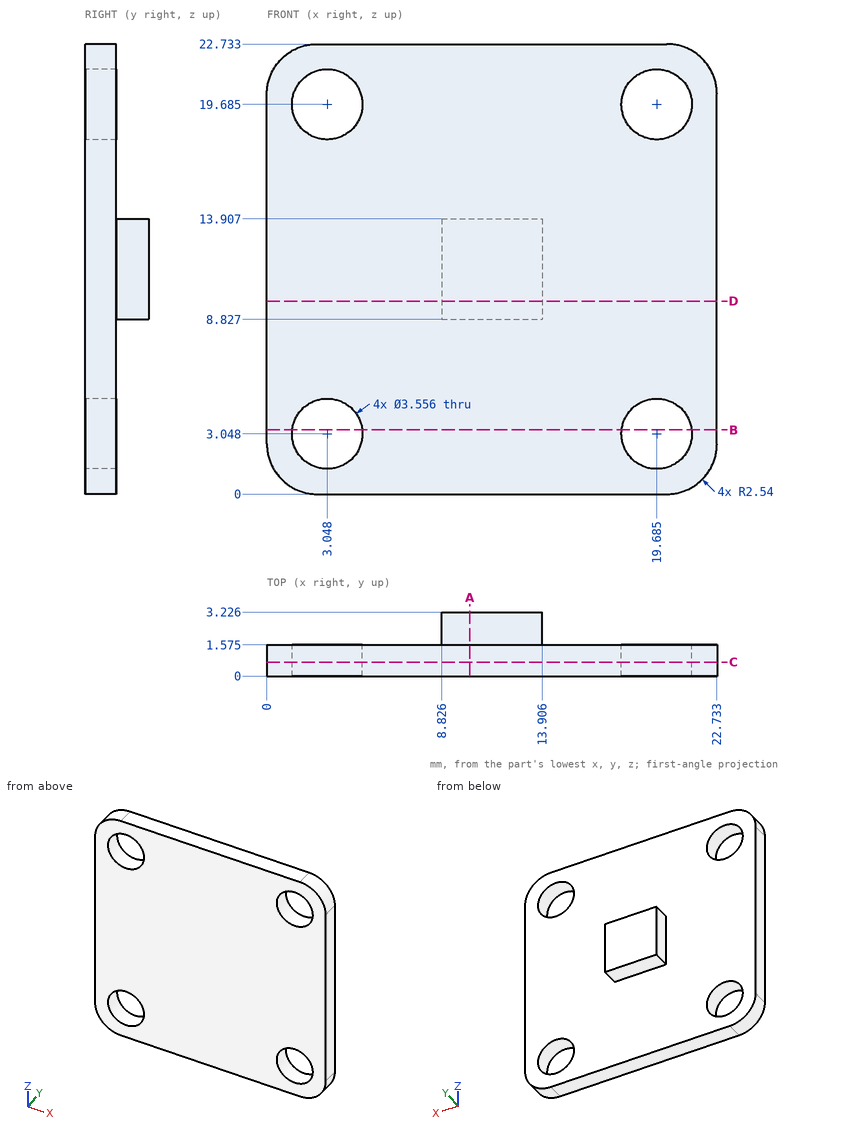
Input: dimensioned drawing with shaded views. Units: mm. Origin: part minimum x, y, z. Coordinates: 2 decimals unless noted, no trailing zeros. Loops run counter-clockwise (first coordinate to the right, second up) from the corner with the lowest first, then second, coordinate; pieces in that order, holes last. Notation, with made-up numbers: M 47.25,-36 L 56.25,-36 A19 ccw 56.25,-13 Z; hole C 43.5,23.25 d6. An arc over 180 degrees is marked long. One line per item, written item: value. Start each with the question number.
1) Pin query (flat end, axial travel): P1, Ø1, axis at x = 11.5, y = 0.5, coming from the -Z side; P2, Ø0.8, axis at y = 2.5, z = 11, coming from the -X side; P3, Ø0.8, axis at y = 2.5, z = 10.5, coming from the +X side. Return the tip coordinate at first contact, or that it passes through.
2) Cut plane D-D (z = 9.75). Return loops of the section in (x, y) (1 decimal).
3) Cut plane B-B (z = 3.25). Return loops of the section in (x, y) (1 decimal).
4) Material intervals for L1, parallel to X at y = 1.4, z = 18.5 (1 decimal); L2, parallel to Y at x = 17.5, z = 11.5 (1 decimal), sorted ascending. Write a range as from..to.
5) Cut plane A-A (x = 10.25). Return loops of the section in (y, z) (1 decimal).
6) Cut plane C-C (y = 0.7). Return loops of the section in (x, z) (1 decimal).
Evaluation:
1. P1: z = 0
1. P2: x = 8.83
1. P3: x = 13.91
2. outline: M 0,0 L 22.7,0 L 22.7,1.6 L 13.9,1.6 L 13.9,3.2 L 8.8,3.2 L 8.8,1.6 L 0,1.6 Z
3. outline: M 0,0 L 1.3,0 L 1.3,1.6 L 0,1.6 Z; M 4.8,0 L 17.9,0 L 17.9,1.6 L 4.8,1.6 Z; M 21.5,0 L 22.7,0 L 22.7,1.6 L 21.5,1.6 Z
4. L1: 0..1.7, 4.4..18.4, 21..22.7
4. L2: 0..1.6
5. outline: M 0,0 L 1.6,0 L 1.6,8.8 L 3.2,8.8 L 3.2,13.9 L 1.6,13.9 L 1.6,22.7 L 0,22.7 Z
6. outline: M 0,2.5 A2.5 ccw 2.5,0 L 20.2,0 A2.5 ccw 22.7,2.5 L 22.7,20.2 A2.5 ccw 20.2,22.7 L 2.5,22.7 A2.5 ccw 0,20.2 Z; hole C 3,3 d3.6; hole C 3,19.7 d3.6; hole C 19.7,3 d3.6; hole C 19.7,19.7 d3.6
